The listing builds one solid part. Answer for the finished solid, in the listing's coordinates (mm). A direction names the side the tool comes from. Round coordinates to 2 decimals unless told otherwise and drop trailing zeros. Write each loop counter-clockwise with the first axis right and the second up, starting at its lowest first coordinate (ties: lowest second). Pieces come first, ordered by that corner, then holes. Notation, with made-up numbers: (-33.5, 53.5) - (18.5, 53.5) arc R19 ccw to (18.5, 65.5) - close; hole circle Ø5 at (-30.5, 67). An arc over 180 degrees is marked (long way). Return JSON: item names as keys, results as strings. Group by question number.
from build123d import *

# Parameters (mm, degrees)
F0_W     = 53
F0_H     = 21
F0_R     = 2.5
F0_W_2   = 15.084836
F0_H_2   = 15
F0_W_3   = 14.984938
F0_W_4   = 13
F0_H_3   = 13
F1_DEPTH = 1.5
F2_DEPTH = 5
F0_R_2   = 1.5
F3_DEPTH = 5


with BuildPart() as f1:
    # F0 (on Top) → F1 (new body)
    with BuildSketch(Plane.XY):
        with Locations((0.118736, -0.1734)):
            Rectangle(F0_W, F0_H)
        with Locations((-23.381264, -7.6734)):
            Circle(F0_R, mode=Mode.SUBTRACT)
        with Locations((-12.518017, -0.1734)):
            Rectangle(F0_W_2, F0_H_2, mode=Mode.SUBTRACT)
        with Locations((23.618736, -7.6734)):
            Circle(F0_R, mode=Mode.SUBTRACT)
        with Locations((12.506826, -0.1734)):
            Rectangle(F0_W_3, F0_H_2, mode=Mode.SUBTRACT)
        with Locations((-23.381264, 7.3266)):
            Circle(F0_R, mode=Mode.SUBTRACT)
        with Locations((23.618736, 7.3266)):
            Circle(F0_R, mode=Mode.SUBTRACT)
        with Locations((-12.518017, -0.1734)):
            Rectangle(F0_W_2, F0_H_2)
        with Locations((-12.5, -0.232354)):
            Rectangle(F0_W_4, F0_H_3, mode=Mode.SUBTRACT)
        with Locations((-12.5, -0.232354)):
            Rectangle(F0_W_4, F0_H_3)
        with Locations((12.506826, -0.1734)):
            Rectangle(F0_W_3, F0_H_2)
        with Locations((12.5, -0.132455)):
            Rectangle(F0_W_4, F0_H_3, mode=Mode.SUBTRACT)
        with Locations((12.5, -0.132455)):
            Rectangle(F0_W_4, F0_H_3)
    extrude(amount=F1_DEPTH)

    # F0 (on Top) → F2 (join)
    with BuildSketch(Plane.XY):
        with Locations((-12.518017, -0.1734)):
            Rectangle(F0_W_2, F0_H_2)
        with Locations((-12.5, -0.232354)):
            Rectangle(F0_W_4, F0_H_3, mode=Mode.SUBTRACT)
        with Locations((12.506826, -0.1734)):
            Rectangle(F0_W_3, F0_H_2)
        with Locations((12.5, -0.132455)):
            Rectangle(F0_W_4, F0_H_3, mode=Mode.SUBTRACT)
    extrude(amount=F2_DEPTH)

    # F0 (on Top) → F3 (join)
    with BuildSketch(Plane.XY):
        with Locations((-23.381264, 7.3266)):
            Circle(F0_R)
        with Locations((-23.381264, 7.3266)):
            Circle(F0_R_2, mode=Mode.SUBTRACT)
        with Locations((-23.381264, -7.6734)):
            Circle(F0_R)
        with Locations((-23.381264, -7.6734)):
            Circle(F0_R_2, mode=Mode.SUBTRACT)
        with Locations((23.618736, -7.6734)):
            Circle(F0_R)
        with Locations((23.618736, -7.6734)):
            Circle(F0_R_2, mode=Mode.SUBTRACT)
        with Locations((23.618736, 7.3266)):
            Circle(F0_R)
        with Locations((23.618736, 7.3266)):
            Circle(F0_R_2, mode=Mode.SUBTRACT)
    extrude(amount=F3_DEPTH)


solid = f1.part
(1) Find section A-A (z = 3.35). State how many separate pieces and enclosed holes the cut face has, plus the area to 3 significant figures.
(2) For faces 1 (the flat face through (19.999, 0, 3)), 2 (the flat face through (25, -9, 5)), 3 (the flat face through (-13, 0, 1.5)), determine the directions among +Z, -Z, +X, -X, +Y, -Y from which every point of the face is accessible in a straight line to the end or side of a thin tool.
(3) Consider line 1 (X direction, y = 2.25, z = 4.6); line 2 (X direction, y = -7.5, z = 0.3); line 3 (X direction, y = 7, z = 3.9). Determine where each line is inside the solid, lowest interval first.
(4) Flat-ended cylindrical pins translate along their axes: pin 1 (1 mm diameter, centred on y = 0.5, z = 2.5, fed in from -X); pin 2 (4 mm diameter, centred on x = -12, y = 0, fed in from +Z); pin 3 (1.8 mm diameter, centred on x = 13.5, z = 3, fed in from -Y); pin 4 (2.5 mm diameter, centred on x = 23.62, y = 7.33, fed in from -Z). Find the tip coordinate at first contact, or state that the pin passes through.
(5) Find section C-C (y = -3.5). Write down the section's boundary in (x, z).
(6) Find section B-B (z = 0.9). Write down the section's boundary in (x, y).
(7) Determine the mould class of faces 4 (the flat face through (5.7, -0.1, 5)), 5 (the flat face through (0, -10.673, 1)), 6 (the cylindrical face through (-23.923, 4.886, 3.226)), 7 (the cylindrical face through (21.63, -9.19, 3.23)) for opening direction Y: +Y half, -Y half, draft (parallel to the pull), parting line (faces both ways), or undercut.
(8) Find section D-D (x = -7.5). Write down the section's boundary in (y, z).
Check sheet entries:
{
 "1": {"separate pieces": "6", "enclosed holes": "6", "area": "163 mm^2"},
 "2": {"face 1": "+Z, +Y, -Y", "face 2": "+Z, +X, -X, +Y, -Y", "face 3": "+Z"},
 "3": {"line 1": "x = -20.06 to -19, -6 to -4.98, 5.01 to 6, 19 to 20", "line 2": "x = -26.38 to -24.87, -21.89 to 22.13, 25.11 to 26.62", "line 3": "x = -25.86 to -24.85, -21.92 to -20.9, -20.06 to -4.98, 5.01 to 20, 21.14 to 22.15, 25.08 to 26.1"},
 "4": {"pin 1": "stops at x = -20.06", "pin 2": "stops at z = 1.5", "pin 3": "stops at y = -7.67", "pin 4": "passes through"},
 "5": {"outline": "(-26.38, 0) - (26.62, 0) - (26.62, 1.5) - (20, 1.5) - (20, 5) - (19, 5) - (19, 1.5) - (6, 1.5) - (6, 5) - (5.01, 5) - (5.01, 1.5) - (-4.98, 1.5) - (-4.98, 5) - (-6, 5) - (-6, 1.5) - (-19, 1.5) - (-19, 5) - (-20.06, 5) - (-20.06, 1.5) - (-26.38, 1.5) - close"},
 "6": {"outline": "(-26.38, -10.67) - (26.62, -10.67) - (26.62, 10.33) - (-26.38, 10.33) - close; hole circle Ø3 at (-23.38, -7.67); hole circle Ø3 at (-23.38, 7.33); hole circle Ø3 at (23.62, -7.67); hole circle Ø3 at (23.62, 7.33)"},
 "7": {"face 4": "draft", "face 5": "-Y half", "face 6": "undercut", "face 7": "undercut"},
 "8": {"outline": "(-10.67, 0) - (10.33, 0) - (10.33, 1.5) - (7.33, 1.5) - (7.33, 5) - (6.27, 5) - (6.27, 1.5) - (-6.73, 1.5) - (-6.73, 5) - (-7.67, 5) - (-7.67, 1.5) - (-10.67, 1.5) - close"}
}
